Model file for the job. Use its own axes, mm. Round coordinates to 2 decimals unless told otherwise and drop trailing zeros. Order: outer loops, then holes, each group sorted by start corner. A loop starts at its lowest first (then second) coordinate and runs counter-clockwise, first axis right, second up. Notation, with made-up numbers: (-13, 32) -> (19, 32) arc R17 ccw to (19, 56) -> close; hole circle Ø2 at (-8.5, -10.5). An arc over 180 degrees is marked (long way). Use CSV: the item, a comma, the result in double quotes.
```python
from build123d import *

# Parameters (mm, degrees)
BOSS_EXTRUDE1_DEPTH      = 38.1
BOSS_EXTRUDE1_DEPTH_BACK = 38.1
SKETCH1_R                = 69.85
SKETCH1_R_2              = 23.412602146
SKETCH1_R_3              = 8.466666667


with BuildPart() as part:
    # Sketch1 → Boss-Extrude1 (new, two sides: drawn at the far end of the back side and taken through both)
    with BuildSketch(Plane.XY.offset(-BOSS_EXTRUDE1_DEPTH_BACK)):
        Circle(SKETCH1_R)
        Circle(SKETCH1_R_2, mode=Mode.SUBTRACT)
        with Locations((-46.631301073, 0)):
            Circle(SKETCH1_R_3, mode=Mode.SUBTRACT)
        with Locations((0, 46.631301073)):
            Circle(SKETCH1_R_3, mode=Mode.SUBTRACT)
        with Locations((46.631301073, 0)):
            Circle(SKETCH1_R_3, mode=Mode.SUBTRACT)
        with Locations((0, -46.631301073)):
            Circle(SKETCH1_R_3, mode=Mode.SUBTRACT)
    extrude(amount=BOSS_EXTRUDE1_DEPTH + BOSS_EXTRUDE1_DEPTH_BACK)


solid = part.part
```
Q1. Cut at D-D (y = -21). Give the cut face in (x, z).
From the geometry:
outline,"(-66.62, -38.1) -> (-10.35, -38.1) -> (-10.35, 38.1) -> (-66.62, 38.1) -> close; (10.35, -38.1) -> (66.62, -38.1) -> (66.62, 38.1) -> (10.35, 38.1) -> close"
Q2. Pin check, flat tips, straight feed: pin 1 (1 mm diameter, centred on x = 32, z = -1, fed in from +Y); pin 2 (8 mm diameter, centred on y = -5.5, z = -12, fed in from +X); pin 3 (1.5 mm diameter, centred on y = 11, z = -28, fed in from -X). Stop position of each tip, or through.
From the geometry:
pin 1,"stops at y = 62.34"
pin 2,"stops at x = 69.83"
pin 3,"stops at x = -69.09"
Q3. Cut at A-A (y = 0). Give the cut face in (x, z), plus the area to 3 significant figures.
From the geometry:
outline,"(-69.85, -38.1) -> (-55.1, -38.1) -> (-55.1, 38.1) -> (-69.85, 38.1) -> close; (-38.16, -38.1) -> (-23.41, -38.1) -> (-23.41, 38.1) -> (-38.16, 38.1) -> close; (23.41, -38.1) -> (38.16, -38.1) -> (38.16, 38.1) -> (23.41, 38.1) -> close; (55.1, -38.1) -> (69.85, -38.1) -> (69.85, 38.1) -> (55.1, 38.1) -> close"
area,"4,500 mm²"
Q4. Cut at C-C (x = -15). Give the cut face in (y, z).
From the geometry:
outline,"(-68.22, -38.1) -> (-17.98, -38.1) -> (-17.98, 38.1) -> (-68.22, 38.1) -> close; (17.98, -38.1) -> (68.22, -38.1) -> (68.22, 38.1) -> (17.98, 38.1) -> close"
Q5. Mould opens along Y. For faces 1 (the flat face through (30, 1, 38.1)), 2 (the cylindrical face through (-1.835, -54.897, -0.533)), 3 (the cylindrical face through (-55.431, -42.503, -0.533)) say: +Y half, -Y half, draft (parallel to the pull), parting line (faces both ways), or undercut.
From the geometry:
face 1,"draft"
face 2,"undercut"
face 3,"parting line"
Q6. Probe line 1 along Y through (x, z) = (0, -7); line 2 along Y through (x, z) = (-4, 31); line 3 along X through (y, z) = (-4.5, 14.5). List the from-to ranges inside material, lowest first.
From the geometry:
line 1,"y = -69.85 to -55.1, -38.16 to -23.41, 23.41 to 38.16, 55.1 to 69.85"
line 2,"y = -69.74 to -54.09, -39.17 to -23.07, 23.07 to 39.17, 54.09 to 69.74"
line 3,"x = -69.7 to -53.8, -39.46 to -22.98, 22.98 to 39.46, 53.8 to 69.7"
